Geometry: final body of the model. Coordinates: model frame, mm. A direction names the side the tool comes from. Round coordinates to 2 decimals unless told otherwise and drop trailing zeros. Write each loop counter-clockwise with the first axis right and the second up, starting at its lowest first coordinate (ties: lowest second). Pieces come first, ordered by that corner, then holes.
from build123d import *

# Parameters (mm, degrees)
ESQUISSE1_W               = 66
ESQUISSE1_H               = 35
BOSS_EXTRU_1_DEPTH        = 70
ESQUISSE2_W               = 54
ESQUISSE2_H               = 35
ENL_V_MAT_EXTRU_2_DEPTH   = 65
ESQUISSE4_W               = 54
ESQUISSE4_H               = 2
BOSS_EXTRU_2_DEPTH        = 30
ESQUISSE5_W               = 6
ESQUISSE5_H               = 51
BOSS_EXTRU_3_DEPTH        = 2
ESQUISSE6_R               = 1
ENL_V_MAT_EXTRU_3_DEPTH   = 10
SYM_TRIE3_COPY_1_SKETCH_R = 1
SYM_TRIE3_COPY_1_DEPTH    = 10
ESQUISSE12_R              = 2.5
ENL_V_MAT_EXTRU_5_DEPTH   = 0.5
ENL_V_MAT_EXTRU_6_DEPTH   = 2
ESQUISSE15_W              = 12
ESQUISSE15_H              = 12
ESQUISSE15_W_2            = 10
ESQUISSE15_H_2            = 15
ENL_V_MAT_EXTRU_8_DEPTH   = 3
ESQUISSE17_W              = 40
ESQUISSE17_H              = 19
ENL_V_MAT_EXTRU_10_DEPTH  = 67
ESQUISSE18_W              = 4
ESQUISSE18_H              = 19
ENL_V_MAT_EXTRU_11_DEPTH  = 30
ESQUISSE20_W              = 67
ESQUISSE20_H              = 5
ENL_V_MAT_EXTRU_13_DEPTH  = 1.5
SYM_TRIE5_COPY_1_SKETCH_W = 67
SYM_TRIE5_COPY_1_SKETCH_H = 5
SYM_TRIE5_COPY_1_DEPTH    = 1.5
ESQUISSE22_W              = 1
ESQUISSE22_H              = 7
ENL_V_MAT_EXTRU_14_DEPTH  = 73


with BuildPart() as part:
    # Esquisse1 → Boss.-Extru.1 (new body)
    with BuildSketch(Plane.XY):
        Rectangle(ESQUISSE1_W, ESQUISSE1_H)
    extrude(amount=BOSS_EXTRU_1_DEPTH)

    # Esquisse2 → Enlèv. mat.-Extru.2 (cut)
    with BuildSketch(Plane.XY.offset(70)):
        Rectangle(ESQUISSE2_W, ESQUISSE2_H)
    extrude(amount=-ENL_V_MAT_EXTRU_2_DEPTH, mode=Mode.SUBTRACT)

    # Esquisse4 → Boss.-Extru.2 (add)
    with BuildSketch(Plane.XY.offset(5)):
        with Locations((0, 16.5)):
            Rectangle(ESQUISSE4_W, ESQUISSE4_H)
    boss_extru_2 = extrude(amount=BOSS_EXTRU_2_DEPTH)

    # Symétrie1: Boss.-Extru.2 across plane
    add(boss_extru_2.mirror(Plane.ZX))

    # Esquisse5 → Boss.-Extru.3 (add)
    with BuildSketch(Plane.XY.offset(70)):
        with Locations((-30, 0)):
            Rectangle(ESQUISSE5_W, ESQUISSE5_H)
    boss_extru_3 = extrude(amount=BOSS_EXTRU_3_DEPTH)

    # Esquisse6 → Enlèv. mat.-Extru.3 (cut)
    with BuildSketch(Plane(origin=(0, 0, 70), x_dir=(-1, 0, 0), z_dir=(0, 0, -1))):
        with Locations((29.930394318, 22)):
            Circle(ESQUISSE6_R)
    enl_v_mat_extru_3 = extrude(amount=-ENL_V_MAT_EXTRU_3_DEPTH, mode=Mode.SUBTRACT)

    # Symétrie2: Enlèv. mat.-Extru.3 across plane
    add(enl_v_mat_extru_3.mirror(Plane.ZX), mode=Mode.SUBTRACT)

    # Symétrie3: Boss.-Extru.3, Enlèv. mat.-Extru.3 across plane
    add(boss_extru_3.mirror(Plane(origin=(0, 0, 0), x_dir=(0, 0, 1), z_dir=(1, 0, 0))))
    add(enl_v_mat_extru_3.mirror(Plane(origin=(0, 0, 0), x_dir=(0, 0, 1), z_dir=(1, 0, 0))), mode=Mode.SUBTRACT)

    # Symétrie3 copy 1 sketch → Symétrie3 copy 1 (cut)
    with BuildSketch(Plane(origin=(0, 0, 70), x_dir=(1, 0, 0), z_dir=(0, 0, -1))):
        with Locations((29.930394318, 22)):
            Circle(SYM_TRIE3_COPY_1_SKETCH_R)
    extrude(amount=-SYM_TRIE3_COPY_1_DEPTH, mode=Mode.SUBTRACT)

    # Esquisse12 → Enlèv. mat.-Extru.5 (cut)
    with BuildSketch(Plane(origin=(0, 0, 0), x_dir=(-1, 0, 0), z_dir=(0, 0, -1))):
        with Locations((0, -12.5)):
            Circle(ESQUISSE12_R)
    extrude(amount=-ENL_V_MAT_EXTRU_5_DEPTH, mode=Mode.SUBTRACT)

    # Esquisse14 → Enlèv. mat.-Extru.6 (cut)
    with BuildSketch(Plane(origin=(0, 0, 0.5), x_dir=(-1, 0, 0), z_dir=(0, 0, -1))):
        with BuildLine():
            Line((0.4, -11.25), (0.4, -13.75))
            ThreePointArc((0.4, -13.75), (0, -14.15), (-0.4, -13.75))
            Line((-0.4, -13.75), (-0.4, -11.25))
            ThreePointArc((-0.4, -11.25), (0, -10.85), (0.4, -11.25))
        make_face()
    extrude(amount=-ENL_V_MAT_EXTRU_6_DEPTH, mode=Mode.SUBTRACT)

    # Esquisse15 → Enlèv. mat.-Extru.8 (cut)
    with BuildSketch(Plane(origin=(0, 0, 0), x_dir=(-1, 0, 0), z_dir=(0, 0, -1))):
        with Locations((1, 3.5)):
            Rectangle(ESQUISSE15_W, ESQUISSE15_H)
        with Locations((-19, 3.5)):
            Rectangle(ESQUISSE15_W, ESQUISSE15_H)
        with Locations((20, 4)):
            Rectangle(ESQUISSE15_W_2, ESQUISSE15_H_2)
    extrude(amount=-ENL_V_MAT_EXTRU_8_DEPTH, mode=Mode.SUBTRACT)

    # Esquisse17 → Enlèv. mat.-Extru.10 (cut, through all)
    with BuildSketch(Plane.ZY.offset(33)):
        with Locations((52, 0)):
            Rectangle(ESQUISSE17_W, ESQUISSE17_H)
    extrude(amount=-ENL_V_MAT_EXTRU_10_DEPTH, mode=Mode.SUBTRACT)

    # Esquisse18 → Enlèv. mat.-Extru.11 (cut)
    with BuildSketch(Plane.XY.offset(32)):
        with Locations((29, 0)):
            Rectangle(ESQUISSE18_W, ESQUISSE18_H)
    enl_v_mat_extru_11 = extrude(amount=-ENL_V_MAT_EXTRU_11_DEPTH, mode=Mode.SUBTRACT)

    # Esquisse20 → Enlèv. mat.-Extru.13 (cut)
    with BuildSketch(Plane.ZY.offset(-27)):
        with Locations((38.5, -13)):
            Rectangle(ESQUISSE20_W, ESQUISSE20_H)
    enl_v_mat_extru_13 = extrude(amount=-ENL_V_MAT_EXTRU_13_DEPTH, mode=Mode.SUBTRACT)

    # Symétrie4: Enlèv. mat.-Extru.13 across plane
    add(enl_v_mat_extru_13.mirror(Plane.ZX), mode=Mode.SUBTRACT)

    # Symétrie5: Enlèv. mat.-Extru.13, Enlèv. mat.-Extru.11 across plane
    add(enl_v_mat_extru_13.mirror(Plane(origin=(0, 0, 0), x_dir=(0, 0, 1), z_dir=(1, 0, 0))), mode=Mode.SUBTRACT)
    add(enl_v_mat_extru_11.mirror(Plane(origin=(0, 0, 0), x_dir=(0, 0, 1), z_dir=(1, 0, 0))), mode=Mode.SUBTRACT)

    # Symétrie5 copy 1 sketch → Symétrie5 copy 1 (cut)
    with BuildSketch(Plane(origin=(-27, 0, 0), x_dir=(0, 0, 1), z_dir=(1, 0, 0))):
        with Locations((38.5, -13)):
            Rectangle(SYM_TRIE5_COPY_1_SKETCH_W, SYM_TRIE5_COPY_1_SKETCH_H)
    extrude(amount=-SYM_TRIE5_COPY_1_DEPTH, mode=Mode.SUBTRACT)

    # Esquisse22 → Enlèv. mat.-Extru.14 (cut, through all)
    with BuildSketch(Plane(origin=(0, 0, 0), x_dir=(-1, 0, 0), z_dir=(0, 0, -1))):
        with Locations((-12.5, 3.5)):
            Rectangle(ESQUISSE22_W, ESQUISSE22_H)
        with Locations((-25.5, 3.5)):
            Rectangle(ESQUISSE22_W, ESQUISSE22_H)
        with Locations((-5.5, 3.5)):
            Rectangle(ESQUISSE22_W, ESQUISSE22_H)
        with Locations((7.5, 3.5)):
            Rectangle(ESQUISSE22_W, ESQUISSE22_H)
    extrude(amount=-ENL_V_MAT_EXTRU_14_DEPTH, mode=Mode.SUBTRACT)


solid = part.part
1) Section A-A on y = -19.5. Output: boundary loops of the cut face in (x, z).
2) Line query: probe 1 along X at (y, z) = (-22, 70.95); probe 2 along Y at (x, z) = (27.5, 64); probe 3 along Y at (x, z) = (-4, 31). Output: solid intervals per line, ascending.
3) Draft query along Y for faces 5 (the flat face through (0, 17, 35)), 6 (the flat face through (30, -25.5, 71)), 7 (the cylindrical face through (-29.14, 21.39, 70.99)), 8 (the flat face through (-30, 25.5, 71)). Return one class per face: pulls with the +Y half, pulls with the -Y half, needs draft (parallel to the pull), parting line crosses it, or undercut.
4) Reachability of faces 1 (the flat face through (25, -1, 1)), 2 (the flat face through (0, -17, 35)), 3 (the flat face through (27, 0, 4)), 4 (the flat face through (25, 3, 4)) from +Z, -Z, +X, -X, +Y, -Y: full face, straight path, thin tool, end or side. Return the list, or none.
5) First-contact query: P1, Ø0.8, axis at x = 12.5, z = 3.5, coming from the -Y side; P2, Ø5, axis at x = -4.5, z = 22, coming from the +Y side; P3, Ø0.6, axis at x = -11.5, y = -16.5, coming from the +Z side. Flat tips, straight axial feed; report the tip coordinate or a pass-through.
6) Section C-C on y = 22. Output: boundary loops of the cut face in (x, z).
7) Section B-B on z = 49. State how many separate pieces and enclosed holes the cut face has, plus the area to 3 significant figures.
8) Section D-D on z = 11. Output: boundary loops of the cut face in (x, y).
Filled in:
1. outline: (-33, 70) - (-27, 70) - (-27, 72) - (-33, 72) - close; (27, 70) - (33, 70) - (33, 72) - (27, 72) - close
2. probe 1: x = -33 to -30.93, -28.93 to -27, 27 to 28.93, 30.93 to 33
2. probe 2: y = -17.5 to -15.5, -10.5 to -9.5, 9.5 to 10.5, 15.5 to 17.5
2. probe 3: y = -17.5 to -15.5, 15.5 to 17.5
3. face 5: needs draft
3. face 6: pulls with the -Y half
3. face 7: undercut
3. face 8: pulls with the +Y half
4. face 1: -Z
4. face 2: +Z, +Y, -Y
4. face 3: +Z
4. face 4: +Z, -Z
5. P1: stops at y = -17.5
5. P2: stops at y = 17.5
5. P3: stops at z = 35
6. outline: (-33, 70) - (-30.93, 70) - (-30.93, 72) - (-33, 72) - close; (-28.93, 70) - (-27, 70) - (-27, 72) - (-28.93, 72) - close; (27, 70) - (28.93, 70) - (28.93, 72) - (27, 72) - close; (30.93, 70) - (33, 70) - (33, 72) - (30.93, 72) - close
7. separate pieces: 4
7. enclosed holes: 0
7. area: 162 mm2
8. outline: (-33, -17.5) - (33, -17.5) - (33, 17.5) - (-33, 17.5) - close; hole (-31, -9.5) - (-27, -9.5) - (-27, -10.5) - (-28.5, -10.5) - (-28.5, -15.5) - (28.5, -15.5) - (28.5, -10.5) - (27, -10.5) - (27, -9.5) - (31, -9.5) - (31, 9.5) - (27, 9.5) - (27, 10.5) - (28.5, 10.5) - (28.5, 15.5) - (-28.5, 15.5) - (-28.5, 10.5) - (-27, 10.5) - (-27, 9.5) - (-31, 9.5) - close
